Part print with two shaded views. Sizes in mm from the minimum x, y, z corner. Round coordinates to 2 decimals unless told otherwise and drop trailing zeros. Order: outer loops, then holes, each group sorted by start corner. A loop starts at its lowest first (then second) coordinate and runs counter-clockwise, first axis right, second up. Notation, with made-up numbers: M -11.75,-22.75 L 32.25,-22.75 A37 ccw 32.25,15.25 Z; hole C 33,-18 d1. An arc over 180 degrees is marked long. Put each result on its own line as item: value.
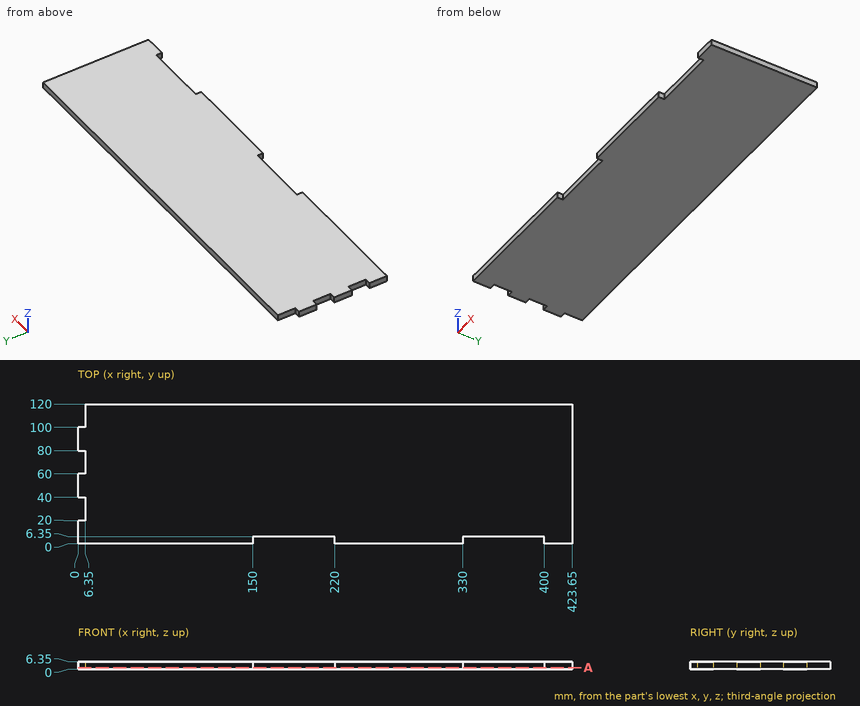
Item 1: Band-saw the part on A-A on z = 1.5. Give the cut face in (x, y), and give its area (3 significant figures).
Answers below:
outline: M 0,0 L 150,0 L 150,6.35 L 220,6.35 L 220,0 L 330,0 L 330,6.35 L 400,6.35 L 400,0 L 423.65,0 L 423.65,120 L 6.35,120 L 6.35,100 L 0,100 L 0,80 L 6.35,80 L 6.35,60 L 0,60 L 0,40 L 6.35,40 L 6.35,20 L 0,20 Z
area: 49,600 mm²
Item 2: Pin check, flat tips, straight feed: P1, Ø3, axis at y = 111.5, z = 3, coming from the -X side; P2, Ø1.9, axis at x = 2.5, z = 3.5, coming from the +Y side; P3, Ø1.9, axis at x = 363, z = 3, coming from the -Y side. Stop position of each tip, or through.
Answers below:
P1: x = 6.35
P2: y = 100
P3: y = 6.35
Item 3: Probe line 1 along X through (y, z) = (37, 2); line 2 along Y through (x, z) = (365, 3). List the from-to ranges inside material, lowest first. Write a range as [from, to].
Answers below:
line 1: [6.35, 423.65]
line 2: [6.35, 120]
